```python
from build123d import *

# Parameters (mm, degrees)
F1_DEPTH = 292.1
F3_DEPTH = 611.632


with BuildPart() as f1:
    # F0 (on Top) → F1 (new body, symmetric)
    with BuildSketch(Plane.XY):
        Polygon((-60.325, 60.325), (-60.325, -60.325), (60.325, -60.325), (60.325, -41.275), (-41.275, -41.275), (-41.275, 60.325), align=None)
    extrude(amount=F1_DEPTH, both=True)

    # F2 (on face) → F3 (cut)
    with BuildSketch(Plane.XY.offset(292.1)):
        with BuildLine():
            ThreePointArc((-47.767103, -50.8), (-47.997968, -49.63936), (-48.655418, -48.655418))
            Line((-48.655418, -48.655418), (-52.944582, -52.944582))
            ThreePointArc((-52.944582, -52.944582), (-49.63936, -53.602032), (-47.767103, -50.8))
        make_face()
        with BuildLine():
            Line((-52.944582, -52.944582), (-48.655418, -48.655418))
            ThreePointArc((-48.655418, -48.655418), (-52.944582, -48.655418), (-52.944582, -52.944582))
        make_face()
    extrude(amount=-F3_DEPTH, mode=Mode.SUBTRACT)


solid = f1.part
```
Geometry check sheet. Reference: the model listing, model coordinates, mm. A direction names the side the tool comes from. Coordinates: 2 decimals unless noted, no trailing zeros. Loops run counter-clockwise (first coordinate to the right, second up) from the corner with the lowest first, then second, coordinate; pieces in that order, holes last.
Item 1: Access from +Z, -Z, +X, -X, +Y, -Y to the whole of each face (thin tool, end or side, straight path). Record for faces 1 (the face through (10, -41.275, 4)), 2 (the face through (-27, -44, 292.1)).
Item 2: Thickness scan on line 1 (X direction, y = -19.5, z = 228) (3 decimals); line 2 (Y direction, x = -52, z = -234) (3 decimals). Record the ranges inside material, lowest first.
Item 3: Sectioned sample at A-A, the plane z = 91.5. Record the boundary of the cut face in (x, y) (3 decimals).
Item 4: Sectioned sample at B-B, the plane x = -16. Record the boundary of the cut face in (y, z) (3 decimals), then the cut area to 3 significant figures.
Item 5: Go/stop test with a flat-tipped pin: pin 1 Ø12 at (x, z) = (17, -24.5) entering from +Y (3 decimals). Record where the tip stops, or that it passes through.
Check result:
1. face 1: +Z, -Z, +X, +Y
1. face 2: +Z, +X, -X, +Y, -Y
2. line 1: x = -60.325 to -41.275
2. line 2: y = -60.325 to -53.585, -48.015 to 60.325
3. outline: (-60.325, -60.325) - (60.325, -60.325) - (60.325, -41.275) - (-41.275, -41.275) - (-41.275, 60.325) - (-60.325, 60.325) - close; hole (-52.945, -52.945) arc R3.033 ccw to (-47.767, -50.8) arc R3.033 ccw to (-48.655, -48.655) arc R3.033 ccw to start
4. outline: (-60.325, -292.1) - (-41.275, -292.1) - (-41.275, 292.1) - (-60.325, 292.1) - close
4. area: 11,100 mm2
5. pin 1: stops at y = -41.275
